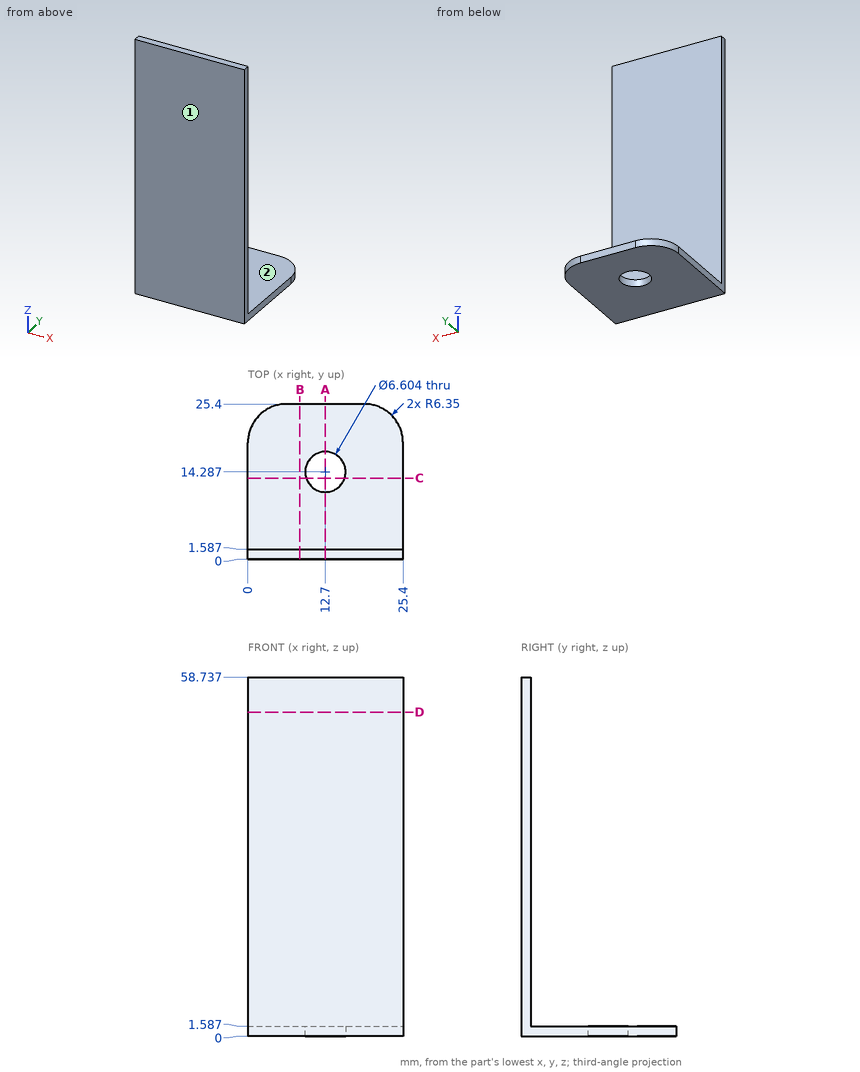
Study the drawing (mm; zero at the part's minimum x, y, z) and answer. A direction names the side the tool comes from. Give positions to 0.01 mm unless a question says otherwise; leave off trailing zeros. Loops run counter-clockwise (first coordinate to the right, second up) from the corner with the lowest first, then second, coordinate; pieces in that order, holes last. Notation, with made-up numbers: (-14, 47.25) -> (-3, 47.25) arc R32 cw to (-3, 81.25) -> close; hole circle Ø1 at (17.25, 33.5). An arc over 180 degrees is marked (long way). Write item = value, one per line. Start each with the question number.
(1) Which of the six approach directions +Z, -Z, +X, -X, +Y, -Y give full straight-line access (tool end or side, diameter ignored) to the marked faces 1 and 2?
(2) Find section B-B on x = 8.5. Give the vertices of the cut face in (y, z).
(3) Find section C-C on y = 13.25. Give the vertices of the cut face in (x, z) (1 decimal).
(4) Find section D-D on z = 53. Give the vertices of the cut face in (x, y).
(5) Given pin 1 Ø5 at (y, z) = (3, 52) entering from -X; pin 2 Ø10 at (y, z) = (22, 9.5) entering from +X; pin 3 Ø8 at (x, y) = (16, 13.5) entering from +Z, each flat-ended and moving along its own axis, determine where each tip first touches the part or whether it passes through.
(6) Find the intervals of material crossed by probe 1 along Y at (x, z) = (12.7, 0.75) (1 decimal); probe 2 along Z at (x, y) = (20.75, 17), in increasing order. Write a range as from..to.
(7) Find section A-A on x = 12.7. Give the vertices of the cut face in (y, z) (1 decimal).
From the geometry:
q1.face_1 = +Z, -Z, +X, -X, -Y
q1.face_2 = +Z, +X, -X, +Y
q2.outline = (0, 0) -> (25.4, 0) -> (25.4, 1.59) -> (1.59, 1.59) -> (1.59, 58.74) -> (0, 58.74) -> close
q3.outline = (0, 0) -> (9.6, 0) -> (9.6, 1.6) -> (0, 1.6) -> close; (15.8, 0) -> (25.4, 0) -> (25.4, 1.6) -> (15.8, 1.6) -> close
q4.outline = (0, 0) -> (25.4, 0) -> (25.4, 1.59) -> (0, 1.59) -> close
q5.pin_1 = 0
q5.pin_2 = through
q5.pin_3 = 1.59
q6.probe_1 = 0..11, 17.6..25.4
q6.probe_2 = 0..1.59
q7.outline = (0, 0) -> (11, 0) -> (11, 1.6) -> (1.6, 1.6) -> (1.6, 58.7) -> (0, 58.7) -> close; (17.6, 0) -> (25.4, 0) -> (25.4, 1.6) -> (17.6, 1.6) -> close
